Check sheet for the drawn part. Datum: minimum x, y, z corner. Units: mm. A direction names the side the tool comes from. Round coordinates to 2 decimals unless told otherwise and drop trailing zeros. Loops run counter-clockwise (first coordinate to the right, second up) from the corner with the lowest first, then second, coordinate; pieces in that order, holes last. Notation, with made-up numbers: (27, -10) - (57, -10) arc R20 ccw to (57, -3) - close; hole circle Ø8 at (80.25, 3). An arc over 180 degrees is marked (long way). Use CSV: the item, a comma, the result in double quotes.
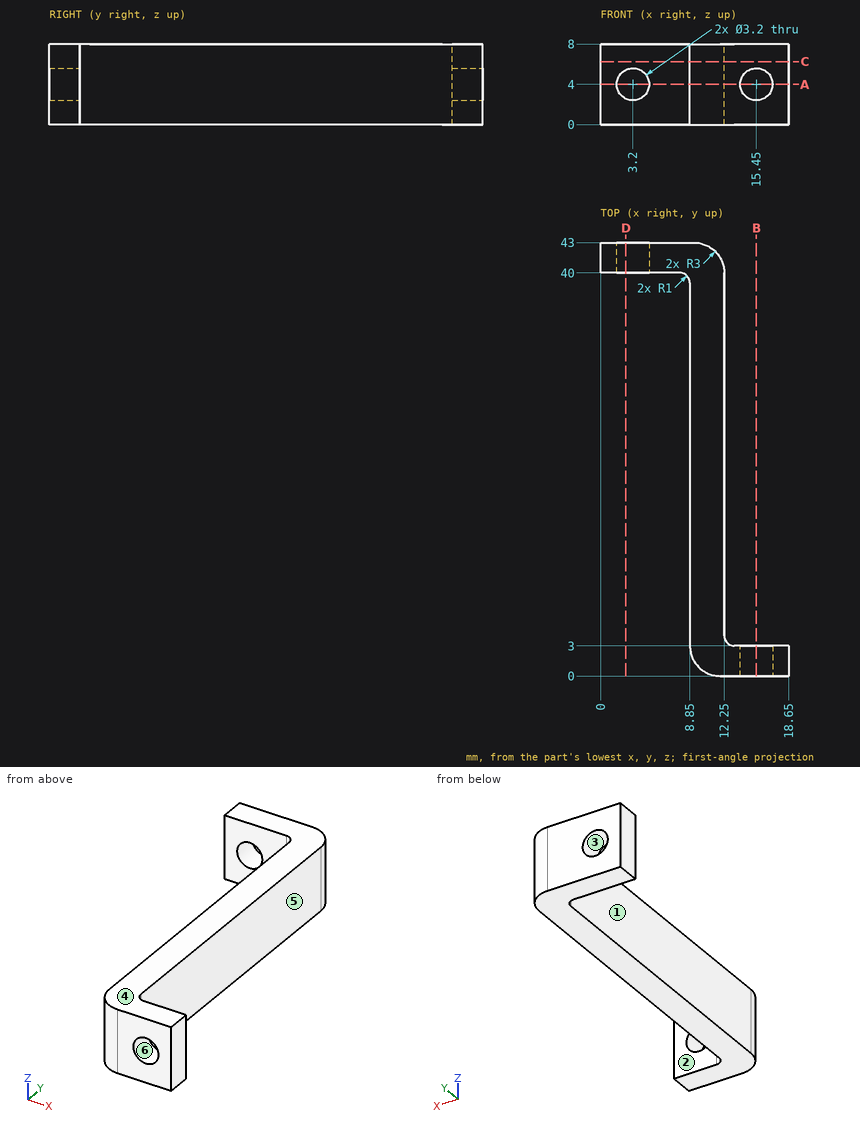
1) Cross-section at D-D, the plane x = 2.5. Record the cut outline in (y, z), then the cut area to 3 significant figures.
Returned:
outline,"(40, 0) - (43, 0) - (43, 2.56) - (40, 2.56) - close; (40, 5.44) - (43, 5.44) - (43, 8) - (40, 8) - close"
area,"15.4 mm²"
2) Mould release check, pull along X, two halves, no side actions. Record for the marked faces 4, 5 and 6: +X half, -X half, draft (parallel to the pull), parting line (faces both ways), or undercut.
Returned:
face 4,"draft"
face 5,"+X half"
face 6,"undercut"
3) Access from +Z, -Z, +X, -X, +Y, -Y to the whole of each face (thin tool, end or side, straight path). Record for the marked faces 1, 2 and 3.
Returned:
face 1,"+Z, -Z, -X, -Y"
face 2,"+Z, -Z, +X, +Y"
face 3,"+Y, -Y"
4) Thickness scan on probe 1 along X at (y, z) = (12, 3.25); probe 2 along X at (y, z) = (1.7, 4); probe 3 along Z at (x, y) = (15.45, 2.25). Record the ranges inside material, lowest first. Write a range as [from, to].
Returned:
probe 1,"x = [8.85, 12.25]"
probe 2,"x = [9.15, 13.85], [17.05, 18.65]"
probe 3,"z = [0, 2.4], [5.6, 8]"
5) Cross-section at B-B, the plane x = 15.45. Record the cut outline in (y, z), then the cut area to 3 significant figures.
Returned:
outline,"(0, 0) - (3, 0) - (3, 2.4) - (0, 2.4) - close; (0, 5.6) - (3, 5.6) - (3, 8) - (0, 8) - close"
area,"14.4 mm²"
6) Gauge pin test, flat ends, axial feed: pin 1 Ø2.5 at (x, z) = (15, 2) entering from +Y; pin 2 Ø1.5 at (y, z) = (11.5, 4) entering from -X. Record the tip position at first contact, or that the pin passes through.
Returned:
pin 1,"stops at y = 3"
pin 2,"stops at x = 8.85"
7) Cross-section at A-A, the plane z = 4. Record the cut outline in (x, y), then the cut area to 3 significant figures.
Returned:
outline,"(0, 40) - (1.6, 40) - (1.6, 43) - (0, 43) - close; (4.8, 40) - (7.85, 40) arc R1 cw to (8.85, 39) - (8.85, 3) arc R3 ccw to (11.85, 0) - (13.85, 0) - (13.85, 3) - (13.25, 3) arc R1 cw to (12.25, 4) - (12.25, 40) arc R3 ccw to (9.25, 43) - (4.8, 43) - close; (17.05, 0) - (18.65, 0) - (18.65, 3) - (17.05, 3) - close"
area,"169 mm²"
8) Cross-section at C-C, the plane z = 6.25. Record the cut outline in (x, y).
Returned:
outline,"(0, 40) - (7.85, 40) arc R1 cw to (8.85, 39) - (8.85, 3) arc R3 ccw to (11.85, 0) - (18.65, 0) - (18.65, 3) - (13.25, 3) arc R1 cw to (12.25, 4) - (12.25, 40) arc R3 ccw to (9.25, 43) - (0, 43) - close"
